Autodesk Inventor part; units mm, degrees
ref_plane "工作平面1" through (10, 19, 0) normal (-0.4333, -0.6373, -0.6373) x (0.8269, 0, -0.5623)
ref_plane "YZ Plane" through (0, 0, 0) normal (1, 0, 0) x (0, 1, 0)
ref_plane "XZ Plane" through (0, 0, 0) normal (0, 1, 0) x (-1, 0, 0)
sketch "草圖1" plane through (0, 0, 0) normal (0, 1, 0) x (-1, 0, 0)
  line L0 (0, 0) -> (-60, 0)
  line L1 (-60, 0) -> (-60, -44)
  line L2 (-60, -44) -> (0, -44)
  line L3 (0, -44) -> (0, 0)
  dimension "d0" = 60
  dimension "d1" = 44
extrude "擠出1" add sketch "草圖1" along normal mid plane 38
sketch "草圖2" plane through (0, 19, 0) normal (0, 1, 0) x (1, 0, 0)
  line L0 (0, 0) -> (60, 0)
  line L1 (10, 0) -> (60, 14)
  line L2 (60, 0) -> (60, 44)
  dimension "d4" = 10
  dimension "d5" = 30
extrude "擠出2" cut sketch "草圖2" against normal blind 40
sketch "草圖3" plane through (60, -19, -44) normal (1, 0, 0) x (0, 0, -1)
  line L0 (-30, 18) -> (-10, 38)
  line L1 (0, 38) -> (-44, 38)
  line L2 (-30, 38) -> (-30, 0)
  point P0 (-44, 19)
  dimension "d8" = 20
  dimension "d9" = 20
ref_plane "工作平面1" through (10, 19, 0) normal (-0.4333, -0.6373, -0.6373) x (0.8269, 0, -0.5623)
sketch "草圖4" plane through (10, 19, 0) normal (-0.4333, -0.6373, -0.6373) x (0.8269, 0, -0.5623)
  line L0 (-15.1543, -12.3218) -> (93.717, -12.3218)
  line L1 (93.717, -12.3218) -> (93.717, 28.8166)
  line L2 (93.717, 28.8166) -> (-15.1543, 28.8166)
  line L3 (-15.1543, 28.8166) -> (-15.1543, -12.3218)
  point P0 (-8.2693, 11.0588)
extrude "擠出3" cut sketch "草圖4" against normal blind 40
mirror "鏡射1" about plane through (0, 0, 0) normal (0, 1, 0) of "擠出3"
properties part number "43"
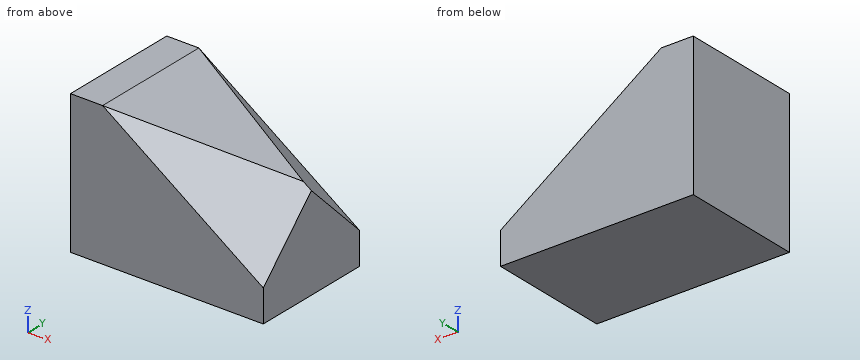
Input: part model. Units: mm. Frame: model coordinates. Round coordinates to 2 decimals unless told otherwise and drop trailing zeros. Write each loop counter-clockwise with the first axis right and the second up, starting at its lowest first coordinate (ties: lowest second). Pieces come first, ordered by that corner, then holes. Notation, with made-up numbers: M -30.5,21 L 1.5,21 A28 ccw 1.5,59 Z; hole C -37.5,-28.5 d10. An arc over 180 degrees is marked long. Write each question's results on one line, items separated by ' | '.
Q1. Pin query (flat end, axial travel): P1, Ø1, axis at x = 18.5, y = 15, coming from the +Z side; P2, Ø6, axis at x = 14.5, y = 8, coming from the +Z side; P3, Ø10, axis at x = 28.5, y = -2.5, coming from the +Z side. Return the tip coordinate at first contact, or that it passes through.
Results:
P1: stops at z = -2.24 | P2: stops at z = -0.42 | P3: stops at z = -3.78
Q2. Line query: line 1 along Z through (x, y) = (19, -15.5); line 2 along X through (y, z) = (6, -14.5); line 3 along X through (y, z) = (-12, -8.5). Output: solid intervals per line, ascending.
Results:
line 1: z = -44 to -2.62 | line 2: x = 0 to 50.44 | line 3: x = 0 to 32.79
Q3. Section query B-B (x = 38). Return loops of the section in (y, z).
Results:
outline: M -19,-44 L 19,-44 L 19,-19.04 L 7.8,-7.84 L -7.8,-7.84 L -19,-19.04 Z
Q4. Section query A-A (y = 11). Return loops of the section in (x, z).
Results:
outline: M 0,-44 L 60,-44 L 60,-26 L 30,-5.6 L 10,0 L 0,0 Z
